from build123d import *

# Parameters (mm, degrees)
SKETCH1_RX           = 24.5
SKETCH1_RY           = 16
BASE_DEPTH           = 1
SKETCH2_R            = 14
SUPORTE_ESFERA_DEPTH = 20
FILLET1_R            = 14
SKETCH3_R            = 2
FUROS_BASE_DEPTH     = 2


with BuildPart() as part:
    # Sketch1 → Base (new body)
    with BuildSketch(Plane(origin=(0, 0, 0), x_dir=(1, 0, 0), z_dir=(0, 1, 0))):
        with Locations(Location((0, 0), (0, 0, 180))):
            Ellipse(SKETCH1_RX, SKETCH1_RY)
    extrude(amount=BASE_DEPTH)

    # Sketch2 → Suporte-esfera (add)
    with BuildSketch(Plane(origin=(0, 1, 0), x_dir=(1, 0, 0), z_dir=(0, 1, 0))):
        Circle(SKETCH2_R)
    extrude(amount=SUPORTE_ESFERA_DEPTH)

    # Fillet1
    fillet1_edges = [part.edges().sort_by_distance(p)[0] for p in [
        (-14, 21, 0),
    ]]
    fillet(fillet1_edges, radius=FILLET1_R)

    # Sketch3 → Furos-base (cut, through all)
    with BuildSketch(Plane(origin=(0, 1, 0), x_dir=(1, 0, 0), z_dir=(0, 1, 0))):
        with Locations((-19, 0)):
            Circle(SKETCH3_R)
        with Locations((19, 0)):
            Circle(SKETCH3_R)
    extrude(amount=-FUROS_BASE_DEPTH, mode=Mode.SUBTRACT)


solid = part.part
CAD build for the part. Positions are in the model's coordinates, mm. A direction names the side the tool comes from. Give positions to 0.01 mm unless a question says otherwise; leave off trailing zeros. Write each loop counter-clockwise with the first axis right and the second up, starting at its lowest first coordinate (ties: lowest second). Pieces come first, ordered by that corner, then holes. Notation, with made-up numbers: M 86,16 L 93,16 A13 cw 93,31 Z; hole C 68,82 d2. An arc over 180 degrees is marked long. Put each result on its own line as item: value. Start each with the question number.
(1) Band-saw the part on B-B, the plane y = 9.5. Write the cut outline in (x, z), and give its area (3 significant figures).
(2) Probe L1, parallel to X at y = 0.3, z = 0; L2, parallel to Y at x = 15, z = -1.5; L3, parallel to Z at x = -19, y = 0.85. List the from-to ranges inside material, lowest first.
(3) Mould opens along X. For faces 1 (the face through (0, 0, 0)), 2 (the face through (17.4, 0.5, 1.2)), 3 (the face through (12.932, 3.958, 5.362)) say: +X half, -X half, draft (parallel to the pull), parting line (faces both ways), or undercut.
(4) Flat gauge pins, fed straight in: pin 1 Ø1 at (x, z) = (-7.5, 2) entering from +Y; pin 2 Ø10 at (x, y) = (-17, 10) entering from -Z; pin 3 Ø3 at (y, z) = (18, 6.5) entering from -X; pin 4 Ø4 at (x, y) = (-17, 11.5) entering from -Z. Where does each tip first touch, or does it go through?
(5) Band-saw the part on A-A, the plane y = 5.25. Write the cut outline in (x, z), and give its area (3 significant figures).
(6) Which spindle directions (+Z, -Z, +X, -X, +Y, -Y) get a long thin tool onto all of the face, cutting with end or side? Do faces 4 (the face through (-11, 1, -10)), 5 (the face through (-20.6, 0.5, 1.2)). Say none if no direction does.
Response values:
1. outline: C 0,0 d27.55
1. area: 596 mm2
2. L1: x = -24.5 to -21, -17 to 17, 21 to 24.5
2. L2: y = 0 to 1
2. L3: z = -10.1 to -2, 2 to 10.1
3. face 1: draft
3. face 2: undercut
3. face 3: parting line
4. pin 1: stops at y = 18.97
4. pin 2: stops at z = -6.75
4. pin 3: stops at x = -8.3
4. pin 4: passes through
5. outline: C 0,0 d28
5. area: 616 mm2
6. face 4: +Y
6. face 5: +Y, -Y
